Could you check a few things on this model? Use its own coordinates, in mm. Face numbers are marked on the shaded views. A direction names the side the tool comes from. Give positions to 0.01 mm unless a question says otherwise; leave off trailing zeros. Write each loop counter-clockwise with the first axis right and the second up, starting at its lowest first coordinate (ties: lowest second). Pieces come first, ordered by that corner, then holes. Notation, with made-up numbers: (75.25, 23.5) - (132.25, 23.5) arc R22 cw to (132.25, 45.5) - close; hole circle Ø1 at (3, 80). An arc over 180 degrees is marked (long way). Answer as a JSON object with one key per item and string values. Group by question number.
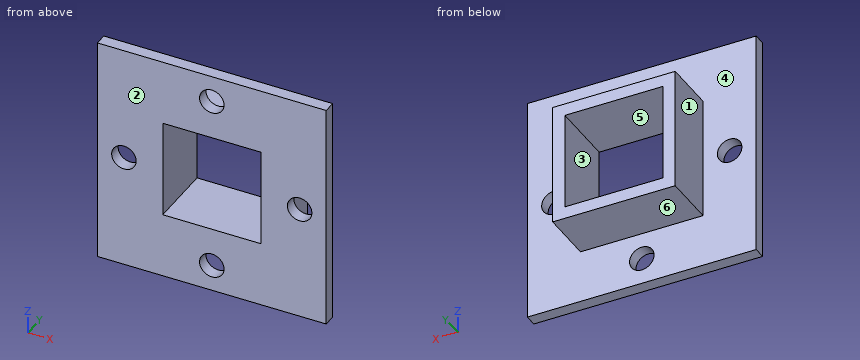
```python
from build123d import *

# Parameters (mm, degrees)
CROQUIS3_W              = 177.8
CROQUIS3_H              = 177.8
CROQUIS3_W_2            = 76.2
CROQUIS3_H_2            = 76.2
SALIENTE_EXTRUIR2_DEPTH = 9.525
CROQUIS4_W              = 95.25
CROQUIS4_H              = 95.25
CROQUIS4_W_2            = 76.2
CROQUIS4_H_2            = 76.2
SALIENTE_EXTRUIR3_DEPTH = 41.275
CROQUIS5_R              = 9.525
CORTAR_EXTRUIR1_DEPTH   = 12


with BuildPart() as part:
    # Croquis3 → Saliente-Extruir2 (new body)
    with BuildSketch(Plane(origin=(0, 0, 0), x_dir=(1, 0, 0), z_dir=(0, 1, 0))):
        Rectangle(CROQUIS3_W, CROQUIS3_H)
        Rectangle(CROQUIS3_W_2, CROQUIS3_H_2, mode=Mode.SUBTRACT)
    extrude(amount=SALIENTE_EXTRUIR2_DEPTH)

    # Croquis4 → Saliente-Extruir3 (add)
    with BuildSketch(Plane(origin=(0, 9.525, 0), x_dir=(1, 0, 0), z_dir=(0, 1, 0))):
        Rectangle(CROQUIS4_W, CROQUIS4_H)
        Rectangle(CROQUIS4_W_2, CROQUIS4_H_2, mode=Mode.SUBTRACT)
    extrude(amount=SALIENTE_EXTRUIR3_DEPTH)

    # Croquis5 → Cortar-Extruir1 (cut)
    with BuildSketch(Plane(origin=(0, 9.525, 0), x_dir=(1, 0, 0), z_dir=(0, 1, 0))):
        with Locations(Location((0, -68.2625, 0), (0, 0, 270))):
            Circle(CROQUIS5_R)
        with Locations(Location((0, 68.2625, 0), (0, 0, 90))):
            Circle(CROQUIS5_R)
        with Locations(Location((-68.2625, 0, 0), (0, 0, 90))):
            Circle(CROQUIS5_R)
        with Locations(Location((68.2625, 0, 0), (0, 0, 270))):
            Circle(CROQUIS5_R)
    extrude(amount=-CORTAR_EXTRUIR1_DEPTH, mode=Mode.SUBTRACT)


solid = part.part
```
(1) For the marked faces 1, 2 and 3, which set-ups out of +Z, -Z, +X, -X, +Y, -Y let a thin tool reach every point of the face, with its end or its side?
(2) I want a section at C-C, the plane z = 0. Please give me the cut outline in (x, y) (1 decimal).
(3) I want a section at A-A, the plane x = 0. Please give me the cut outline in (y, z) (1 decimal).
(4) I need wall thicknesses on L1, parallel to X at y = 3, z = 0; L2, parallel to Z at x = -11, y = 16 (3 decimals). Which ranges of each line are inside material? Lowest first, please.
(5) I want a section at B-B, the plane y = 20.5. Please give me the cut outline in (x, z) (3 decimals).
(6) If we mould it in two halves opening along Z, with no side actions, what happens to the marked faces 4, 5 and 6? For each: +Z half, -Z half, draft (parallel to the pull), parting line (faces both ways), or undercut.
(7) Will these pins go through, and if not, where does the flat tip stop? P1, Ø1, axis at y = 39.5, z = -34.5, coming from the +X side (3 decimals); P2, Ø15, axis at y = 29, z = -12, coming from the -X side (3 decimals); P3, Ø3, axis at x = 37, y = 42, coming from the -Z side (3 decimals); P4, Ø6, axis at y = 28, z = -53.5, coming from the -X side (1 decimal).
(8) I want a section at D-D, the plane x = 31. Please give me the cut outline in (y, z) (3 decimals).
Entries:
{
 "1": {"face 1": "+Z, -Z, -X, +Y", "face 2": "+Z, -Z, +X, -X, -Y", "face 3": "+Y, -Y"},
 "2": {"outline": "(-88.9, 0) - (-77.8, 0) - (-77.8, 9.5) - (-88.9, 9.5) - close; (-58.7, 0) - (-38.1, 0) - (-38.1, 50.8) - (-47.6, 50.8) - (-47.6, 9.5) - (-58.7, 9.5) - close; (38.1, 0) - (58.7, 0) - (58.7, 9.5) - (47.6, 9.5) - (47.6, 50.8) - (38.1, 50.8) - close; (77.8, 0) - (88.9, 0) - (88.9, 9.5) - (77.8, 9.5) - close"},
 "3": {"outline": "(0, -88.9) - (9.5, -88.9) - (9.5, -77.8) - (0, -77.8) - close; (0, -58.7) - (9.5, -58.7) - (9.5, -47.6) - (50.8, -47.6) - (50.8, -38.1) - (0, -38.1) - close; (0, 38.1) - (50.8, 38.1) - (50.8, 47.6) - (9.5, 47.6) - (9.5, 58.7) - (0, 58.7) - close; (0, 77.8) - (9.5, 77.8) - (9.5, 88.9) - (0, 88.9) - close"},
 "4": {"L1": "-88.9 to -77.79, -58.74 to -38.1, 38.1 to 58.74, 77.79 to 88.9", "L2": "-47.625 to -38.1, 38.1 to 47.625"},
 "5": {"outline": "(-47.625, -47.625) - (47.625, -47.625) - (47.625, 47.625) - (-47.625, 47.625) - close; hole (-38.1, -38.1) - (38.1, -38.1) - (38.1, 38.1) - (-38.1, 38.1) - close"},
 "6": {"face 4": "draft", "face 5": "undercut", "face 6": "-Z half"},
 "7": {"P1": "x = 47.625", "P2": "x = -47.625", "P3": "z = -47.625", "P4": "through"},
 "8": {"outline": "(0, -88.9) - (9.525, -88.9) - (9.525, -47.625) - (50.8, -47.625) - (50.8, -38.1) - (0, -38.1) - close; (0, 38.1) - (50.8, 38.1) - (50.8, 47.625) - (9.525, 47.625) - (9.525, 88.9) - (0, 88.9) - close"}
}
